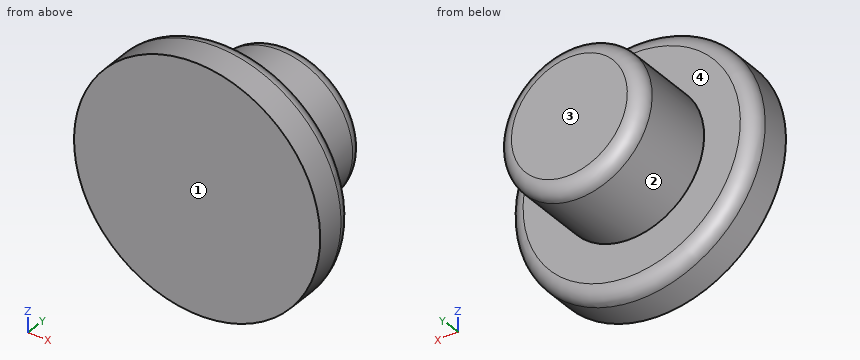
```python
from build123d import *

# Parameters (mm, degrees)
SKETCH1_R           = 8.5
BOSS_EXTRUDE1_DEPTH = 3
FILLET2_R           = 1
SKETCH2_R           = 5
BOSS_EXTRUDE3_DEPTH = 6
FILLET4_R           = 1


with BuildPart() as part:
    # Sketch1 → Boss-Extrude1 (new body)
    with BuildSketch(Plane(origin=(0, 0, 0), x_dir=(1, 0, 0), z_dir=(0, 1, 0))):
        with Locations(Location((-51.120170416, 0, 0), (0, 0, 270))):
            Circle(SKETCH1_R)
    extrude(amount=BOSS_EXTRUDE1_DEPTH)

    # Fillet2
    fillet2_edges = [part.edges().sort_by_distance(p)[0] for p in [
        (-51.120170416, 3, -8.5),
    ]]
    fillet(fillet2_edges, radius=FILLET2_R)

    # Sketch2 → Boss-Extrude3 (add)
    with BuildSketch(Plane(origin=(0, 3, 0), x_dir=(1, 0, 0), z_dir=(0, 1, 0))):
        with Locations(Location((-51.120170416, 0, 0), (0, 0, 270))):
            Circle(SKETCH2_R)
    extrude(amount=BOSS_EXTRUDE3_DEPTH)

    # Fillet4
    fillet4_edges = [part.edges().sort_by_distance(p)[0] for p in [
        (-51.120170416, 9, -5),
    ]]
    fillet(fillet4_edges, radius=FILLET4_R)


solid = part.part
```
Model file for the job. Use its own axes, mm. Face numbers are marked on the shaded views. A direction names the side the tool comes from. Coordinates: 2 decimals unless noted, no trailing zeros. Write each loop counter-clockwise with the first axis right and the second up, starting at its lowest first coordinate (ties: lowest second). Pieces come first, ordered by that corner, then holes. Notation, with made-up numbers: (48.5, 31) - (79.5, 31) arc R31 cw to (79.5, 57) - close; hole circle Ø2 at (74, 62.5). An arc over 180 degrees is marked (long way). Use a Markdown table: item, result. Add a question column.
Item 1: Two-plate mould, pull along Z, no slides. Class the marked faces 1 and 2: pulls with the +Z half, pulls with the -Z half, needs draft (parallel to the pull), parting line crosses it, or undercut.
Item 2: Drill centre lines: line 1 along X through (y, z) = (1.5, 7.5); line 2 along Y through (x, z) = (-47.75, -6.75); line 3 along Z through (x, y) = (-51.25, 1.25). Where is each one in solid material? Low to high.
Item 3: Drop flat-ended pins along their axis: pin 1 (3 mm diameter, centred on x = -50.5, y = 3, fed in from +Z); pin 2 (1.5 mm diameter, centred on x = -50, y = 7, fed in from -Z); pin 3 (5 mm diameter, centred on y = 8, z = 3.5, fed in from +X); pin 4 (3 mm diameter, centred on y = 3.5, z = -3, fed in from -X). Give the stop position or say it passes through.
Item 4: Band-saw the part on B-B, the plane y = 5. Write the cut outline in (x, z), and give its area (3 significant figures).
Item 5: Band-saw the part on C-C, the plane y = 1.25. Write the cut outline in (x, z).
Item 6: 3-axis set-ups, long thin cutter, end or side, ignore diameter. For the marked faces 3 and 4: which of +Z, -Z, +X, -X, +Y, -Y reach the whole face in a straight line?
Item 7: Band-saw the part on A-A, the plane z = 0. Write the cut outline in (x, y).
A:
| question | item | result |
|---|---|---|
| 1 | face 1 | needs draft |
| 1 | face 2 | parting line crosses it |
| 2 | line 1 | x = -55.12 to -47.12 |
| 2 | line 2 | y = 0 to 3 |
| 2 | line 3 | z = -8.5 to 8.5 |
| 3 | pin 1 | stops at z = 8.5 |
| 3 | pin 2 | stops at z = -4.99 |
| 3 | pin 3 | stops at x = -46.22 |
| 3 | pin 4 | stops at x = -59.31 |
| 4 | outline | circle Ø10 at (-51.12, 0) |
| 4 | area | 78.5 mm² |
| 5 | outline | circle Ø17 at (-51.12, 0) |
| 6 | face 3 | +Z, -Z, +X, -X, +Y |
| 6 | face 4 | +Y |
| 7 | outline | (-59.62, 0) - (-42.62, 0) - (-42.62, 2) arc R1 ccw to (-43.62, 3) - (-46.12, 3) - (-46.12, 8) arc R1 ccw to (-47.12, 9) - (-55.12, 9) arc R1 ccw to (-56.12, 8) - (-56.12, 3) - (-58.62, 3) arc R1 ccw to (-59.62, 2) - close |
